Work out the finished part from the listing and answer in its coordinate system (mm). A direction names the side the tool comes from. Give positions to 0.01 mm unless a question says otherwise; leave off trailing zeros. Write each loop counter-clockwise with the first axis right and the second up, starting at its lowest first coordinate (ties: lowest second). Pieces come first, ordered by that corner, then holes. Notation, with made-up numbers: (48, 56) -> (62, 56) arc R21 ccw to (62, 66) -> close; hole circle Ø6 at (-34.5, -37.5). An arc over 180 degrees is marked (long way). Use a Markdown table: item, result. Add a question column.
Q1. Each of these flat-tipped pins is pushed along its axis until it touches: pin 1 Ø2 at (x, y) = (-15.97, 12.66) entering from +Z; pin 2 Ø10 at (x, y) = (-37, -4.5) entering from +Z. Where does it stop, or does it pass through?
Q2. Section A-A, the plane z = 36 is taken. State how many separate pieces and enclosed holes the cut face has, plus the area to 3 significant figures.
Q3. Section B-B, the plane x = 0 is taken. Give the vertices of the cut face in (y, z), plus the area to 3 significant figures.
Q4. For a pull along Y with two mould halves and no side action, classify faces 1 (the face through (0.25, 19.02, 23.29)), 2 (the face through (-4, -34, 47.244)) as pulls with the +Y half, pulls with the -Y half, needs draft (parallel to the pull), parting line crosses it, or undercut.
Q5. Consider line 1 (Y direction, x = 0, z = 3.5); line 2 (Y direction, x = 20, z = 34); line 3 (X direction, y = -31, z = 4). Determine where each line is inside the solid, lowest interval first.
Q6. For faces 3 (the face through (9.075, -16.955, 23.291)), 4 (the face through (0.8, 16.54, 24.58)), determine the directions among +Z, -Z, +X, -X, +Y, -Y from which every point of the face is accessible in a straight line to the end or side of a thin tool.
from build123d import *

# Parameters (mm, degrees)
F0_W     = 95.3876376152
F0_H     = 70.2621340752
F1_DEPTH = 47.244
F3_D     = 2.794
F4_R     = 10.1906585652
F5_DEPTH = 47.244
F6_T     = -2.54


with BuildPart() as f1:
    # F0 (on Top) → F1 (new body)
    with BuildSketch(Plane.XY):
        Rectangle(F0_W, F0_H)
    extrude(amount=F1_DEPTH)

    # F3 (through all)
    with Locations(Plane.XY.offset(47.244)):
        with Locations((-0.0553504175, 20.3824730712), (-15.9701695585, 12.6649893976), (-19.8591252898, -4.5894896111), (-8.7937546256, -18.3879893341), (8.8934926316, -18.3399580419), (19.883758543, -4.4815642772), (15.9011487168, 12.7515387955)):
            Hole(F3_D / 2)

    # F4 (on face) → F5 (cut, through all)
    with BuildSketch(Plane.XY.offset(47.244)):
        Circle(F4_R)
    extrude(amount=-F5_DEPTH, mode=Mode.SUBTRACT)

    # F6
    f6_openings = [f1.faces().sort_by_distance(p)[0] for p in [
        (-46.509101, 0, 47.244),
    ]]
    offset(amount=F6_T, openings=f6_openings)


solid = f1.part
Result set:
| question | item | result |
|---|---|---|
| 1 | pin 1 | passes through |
| 1 | pin 2 | stops at z = 2.54 |
| 2 | separate pieces | 9 |
| 2 | enclosed holes | 9 |
| 2 | area | 1,300 mm2 |
| 3 | outline | (-35.13, 0) -> (-10.19, 0) -> (-10.19, 47.24) -> (-12.73, 47.24) -> (-12.73, 2.54) -> (-32.59, 2.54) -> (-32.59, 47.24) -> (-35.13, 47.24) -> close; (10.19, 0) -> (18.99, 0) -> (18.99, 47.24) -> (16.45, 47.24) -> (16.45, 2.54) -> (12.73, 2.54) -> (12.73, 47.24) -> (10.19, 47.24) -> close; (21.78, 0) -> (35.13, 0) -> (35.13, 47.24) -> (32.59, 47.24) -> (32.59, 2.54) -> (24.32, 2.54) -> (24.32, 47.24) -> (21.78, 47.24) -> close |
| 3 | area | 801 mm2 |
| 4 | face 1 | undercut |
| 4 | face 2 | needs draft |
| 5 | line 1 | y = -35.13 to -32.59, -12.73 to -10.19, 10.19 to 12.73, 16.45 to 18.99, 21.78 to 24.32, 32.59 to 35.13 |
| 5 | line 2 | y = -35.13 to -32.59, -8.42 to -5.87, -3.09 to -0.55, 32.59 to 35.13 |
| 5 | line 3 | x = -47.69 to -45.15, 45.15 to 47.69 |
| 6 | face 3 | +Z, -Z |
| 6 | face 4 | +Z |
